```python
from build123d import *

# Parameters (mm, degrees)
BOSS_EXTRUDE1_DEPTH = 20
FILLET1_R           = 3
SKETCH2_R           = 1.5
CUT_EXTRUDE1_DEPTH  = 20
SKETCH3_R           = 1.5
CUT_EXTRUDE2_DEPTH  = 20


with BuildPart() as part:
    # Sketch1 → Boss-Extrude1 (new body)
    with BuildSketch(Plane.XY):
        Polygon((5, 0), (-17, 0), (-17, 2), (-5, 2), (-5, 10), (-3, 10), (-3, 2), (3, 2), (3, 10), (5, 10), align=None)
    extrude(amount=BOSS_EXTRUDE1_DEPTH)

    # Fillet1
    fillet1_edges = [part.edges().sort_by_distance(p)[0] for p in [
        (4, 10, 0),
        (-17, 1, 0),
        (-4, 10, 0),
        (-4, 10, 20),
        (-17, 1, 20),
        (4, 10, 20),
    ]]
    fillet(fillet1_edges, radius=FILLET1_R)

    # Sketch2 → Cut-Extrude1 (cut)
    with BuildSketch(Plane.ZY.offset(5)):
        with Locations(Location((16, 7, 0), (0, 0, 270))):
            Circle(SKETCH2_R)
        with Locations(Location((4, 7, 0), (0, 0, 270))):
            Circle(SKETCH2_R)
    extrude(amount=-CUT_EXTRUDE1_DEPTH, mode=Mode.SUBTRACT)

    # Sketch3 → Cut-Extrude2 (cut)
    with BuildSketch(Plane(origin=(0, 2, 0), x_dir=(1, 0, 0), z_dir=(0, 1, 0))):
        with Locations(Location((0, -10, 0), (0, 0, 180))):
            Circle(SKETCH3_R)
    extrude(amount=-CUT_EXTRUDE2_DEPTH, mode=Mode.SUBTRACT)


solid = part.part
```
Can you work these out from the model? Positions are in its coordinate system, mm. A direction names the side the tool comes from. Give positions to 0.01 mm unless a question says otherwise; leave off trailing zeros. Loops run counter-clockwise (first coordinate to the right, second up) from the corner with the lowest first, then second, coordinate; pieces in that order, holes last. Notation, with made-up numbers: M 28,46.25 L 74,46.25 A21 cw 74,56.25 Z; hole C 84,44.5 d11. An arc over 180 degrees is marked long. Use one line per item in the form item = value. Start each with the question number.
(1) I'm going to push flat-ended pins straight in: P1, Ø1.8, axis at x = 0, z = 5.5, coming from the +Y side; P2, Ø4, axis at y = 6.5, z = 11.5, coming from the -X side. Where does each tip first touch, or does it pass through?
(2) I want a section at D-D, the plane x = -3.5. Write out the boundary of the cut face in (y, z).
(3) Thinking about a two-plate mould opening in X: for faces 1 (the flat face through (-4, 2, 20)), 2 (the flat face through (-3, 6, 10)), 3 (the cylindrical face through (-16.14, 1.01, 19.1)), 4 (the flat face through (3, 6, 10)), which applies, released by +X, released by -X, zero draft, split by the parting line, or undercut?
(4) I want a section at A-A, the plane y = 3. Write out the boundary of the cut face in (x, z).
(5) I want a section at C-C, the plane x = 0. Write out the boundary of the cut face in (y, z).
(6) Please list where these lines run through material, in increasing order: line 1 (Z direction, x = -4.45, y = 7); line 2 (X direction, y = 7.75, z = 2.25); line 3 (Y direction, x = -15, z = 17).
(7) On a 3-axis mill with a long thin cutter (end or side, diameter ignored), from which of +Z, -Z, +X, -X, +Y, -Y can I reach the whole of each face in a straight line? I mean faces 5 (the flat face through (-5, 6, 10)), 6 (the cylindrical face through (-3.99, 9.14, 0.9)). Say none if no direction works.
(8) I want a section at B-B, the plane z = 16. Write out the boundary of the cut face in (x, y), and give its area (3 significant figures).
Worked out:
q1.P1 = 2
q1.P2 = -5
q2.outline = M 0,0 L 7,0 A3 ccw 10,3 L 10,17 A3 ccw 7,20 L 0,20 Z; hole C 7,4 d3; hole C 7,16 d3
q3.face_1 = zero draft
q3.face_2 = undercut
q3.face_3 = released by -X
q3.face_4 = undercut
q4.outline = M -5,0 L -3,0 L -3,20 L -5,20 Z; M 3,0 L 5,0 L 5,20 L 3,20 Z
q5.outline = M 0,0 L 2,0 L 2,8.5 L 0,8.5 Z; M 0,11.5 L 2,11.5 L 2,20 L 0,20 Z
q6.line_1 = 0 to 2.5, 5.5 to 14.5, 17.5 to 20
q6.line_2 = -5 to -3, 3 to 5
q6.line_3 = 0 to 2
q7.face_5 = +Z, -Z, -X, +Y
q7.face_6 = -Z, +X, -X, +Y
q8.outline = M -17,0 L 5,0 L 5,5.5 L 3,5.5 L 3,2 L -3,2 L -3,5.5 L -5,5.5 L -5,2 L -17,2 Z; M -5,8.5 L -3,8.5 L -3,10 L -5,10 Z; M 3,8.5 L 5,8.5 L 5,10 L 3,10 Z
q8.area = 64.0 mm²
